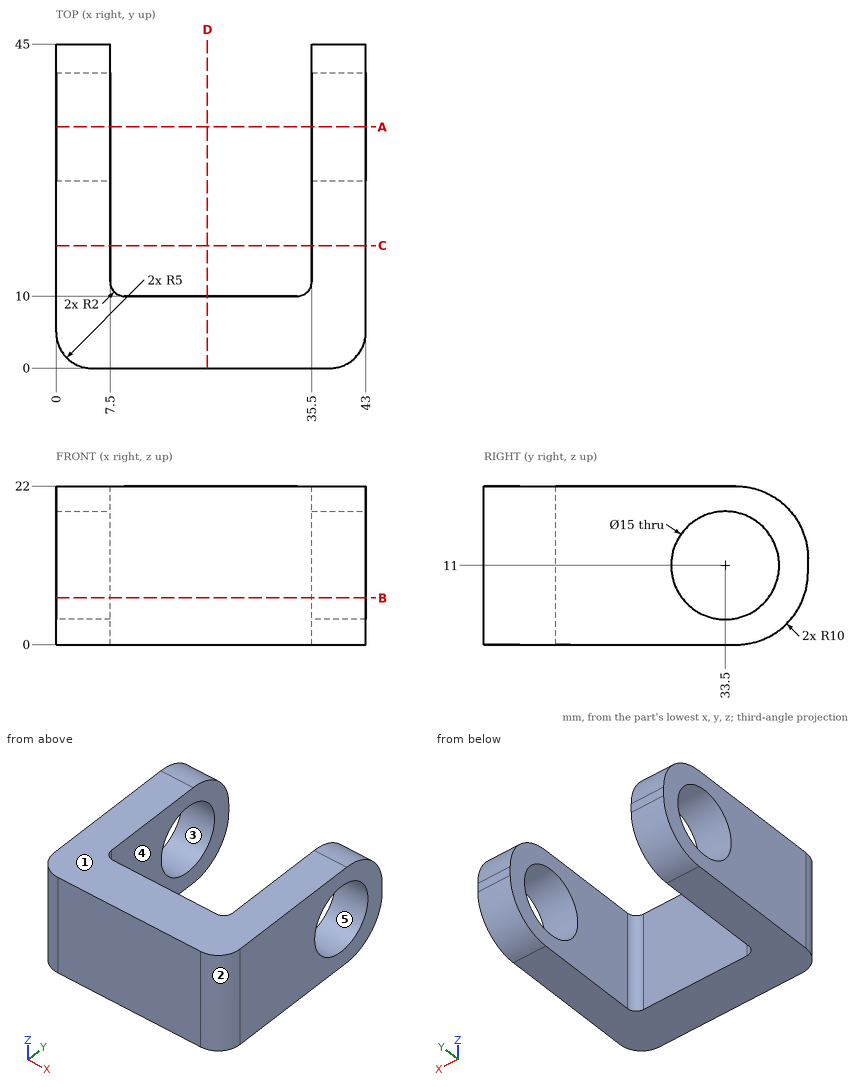
Can you work these out from the drawing? Everything is in mm from the part's minimum corner. A direction names the side the tool comes from. Coordinates: 2 decimals unless noted, no trailing zeros. Order: outer loops, then holes, each group sorted by start corner. A loop starts at its lowest first (then second) coordinate and runs counter-clockwise, first axis right, second up. Notation, with made-up numbers: (47, 16.5) -> (89, 16.5) arc R30 cw to (89, 43.5) -> close; hole circle Ø4 at (43.5, 25.5). An arc over 180 degrees is marked (long way). Use one line per item in the form item = value.
Q1. Will these pins go through, and if not, where does the flat tip stop? P1, Ø9, axis at y = 33.5, z = 11, coming from the +X side; P2, Ø6, axis at x = 18, z = 5, coming from the +Y side.
From the geometry:
P1 = through
P2 = 10
Q2. Imagine slicing it at D-D, the plane x = 21. List the corners of the cut face in (y, z) for me, then the cut area to 3 significant figures.
From the geometry:
outline = (0, 0) -> (10, 0) -> (10, 22) -> (0, 22) -> close
area = 220 mm²
Q3. Imagine slicing it at A-A, the plane y = 33.5. List the corners of the cut face in (x, z) for me, then the cut area to 3 significant figures.
From the geometry:
outline = (0, 0) -> (7.5, 0) -> (7.5, 3.5) -> (0, 3.5) -> close; (0, 18.5) -> (7.5, 18.5) -> (7.5, 22) -> (0, 22) -> close; (35.5, 0) -> (43, 0) -> (43, 3.5) -> (35.5, 3.5) -> close; (35.5, 18.5) -> (43, 18.5) -> (43, 22) -> (35.5, 22) -> close
area = 105 mm²
Q4. Imagine slicing it at B-B, the plane z = 6.5. List the corners of the cut face in (x, y) for me.
From the geometry:
outline = (0, 5) arc R5 ccw to (5, 0) -> (38, 0) arc R5 ccw to (43, 5) -> (43, 27.5) -> (35.5, 27.5) -> (35.5, 12) arc R2 cw to (33.5, 10) -> (9.5, 10) arc R2 cw to (7.5, 12) -> (7.5, 27.5) -> (0, 27.5) -> close; (0, 39.5) -> (7.5, 39.5) -> (7.5, 44.37) -> (0, 44.37) -> close; (35.5, 39.5) -> (43, 39.5) -> (43, 44.37) -> (35.5, 44.37) -> close
Q5. We'd pull the mould along Y, two halves only. Please class the marked faces 1, 2 and 3: released by +Y, released by -Y, zero draft, split by the parting line, or undercut.
From the geometry:
face_1 = zero draft
face_2 = released by -Y
face_3 = undercut
Q6. I need wall thicknesses on L1, parallel to Y at x = 6.5, z = 11; L2, parallel to X at y = 24, z = 2; L3, parallel to Y at x = 3.5, z = 11.75. Which ranges of each line are inside material? Lowest first, please.
From the geometry:
L1 = 0 to 26, 41 to 45
L2 = 0 to 7.5, 35.5 to 43
L3 = 0.23 to 26.04, 40.96 to 45
Q7. Imagine slicing it at C-C, the plane y = 17. List the corners of the cut face in (x, z) for me.
From the geometry:
outline = (0, 0) -> (7.5, 0) -> (7.5, 22) -> (0, 22) -> close; (35.5, 0) -> (43, 0) -> (43, 22) -> (35.5, 22) -> close
Q8. Which directions (+Z, -Z, +X, -X, +Y, -Y) give clear straight access to the entire face, cutting with the end or side of a thin tool? Please do the marked faces 4 and 5.
From the geometry:
face_4 = +Z, -Z, +Y
face_5 = +X, -X
